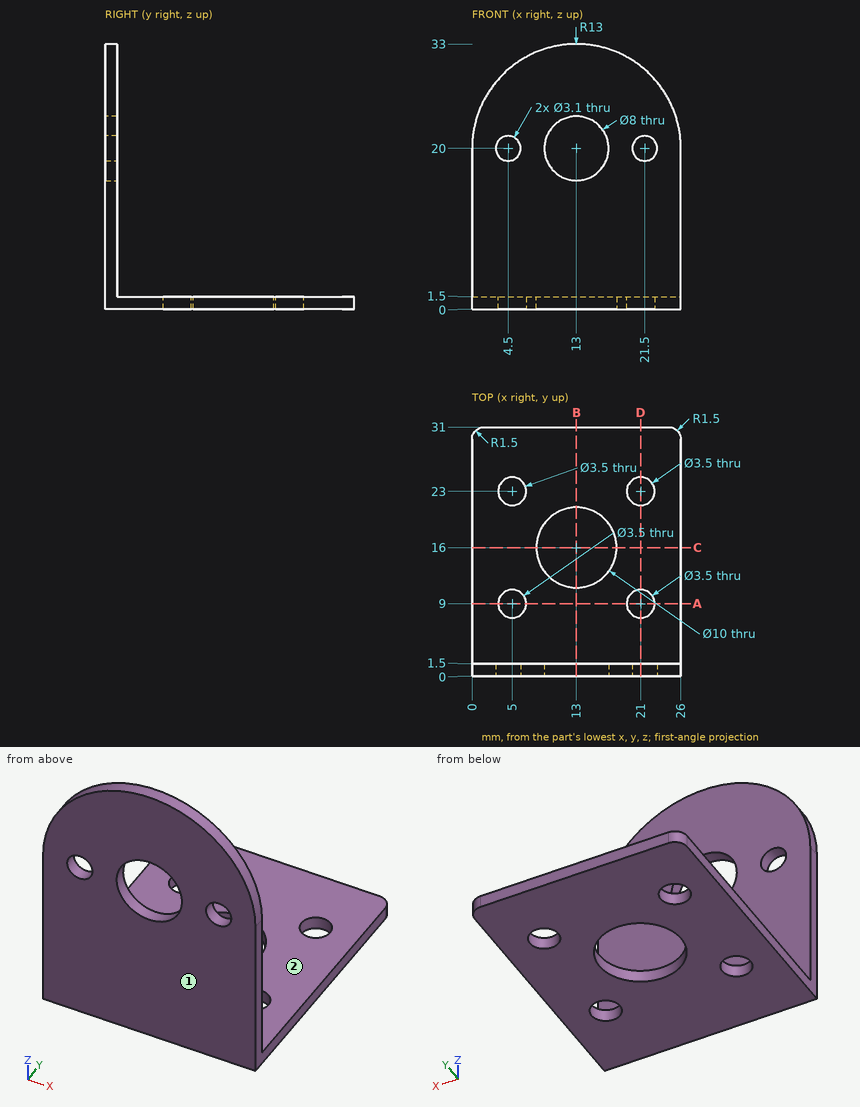
Here's the drawing with two shaded views (mm, measured from the low corner). I have some questions. A direction names the side the tool comes from. Coordinates: 2 decimals unless noted, no trailing zeros. Order: outer loops, then holes, each group sorted by start corner. A loop starts at its lowest first (then second) coordinate and runs counter-clockwise, first axis right, second up. Notation, with made-up numbers: (28, 56) - (34, 56) arc R34 ccw to (34, 94) - close; hole circle Ø8 at (44, 74). An arc over 180 degrees is marked (long way). Answer in a Markdown table with one row per item. Add a question column.
(1) If we section it at D-D, the plane x = 21: Please give me the cut outline in (y, z), then the cut area to 3 significant figures.
(2) I need wall thicknesses on L1, parallel to Y at x = 21, z = 1.2; L2, parallel to X at y = 0.5, z = 20; L3, parallel to Z at x = 12.5, y = 28. Which ranges of each line are inside material? Lowest first, please.
(3) On a 3-axis mill with a long thin cutter (end or side, diameter ignored), from which of +Z, -Z, +X, -X, +Y, -Y can I reach the whole of each face in a straight line? I mean the marked faces 1 and 2. Say none if no direction works.
(4) Will these pins go through, and if not, where does the flat tip stop? pin 1 (3 mm diameter, centred on x = 4, z = 19, fed in from +Y); pin 2 (4 mm diameter, centred on x = 21, y = 23, fed in from +Z).
(5) If we section it at C-C, the plane y = 16: Please give me the cut outline in (x, z), then the cut area to 3 significant figures.
(6) If we section it at B-B, the plane x = 13: Please give me the cut outline in (y, z), then the cut area to 4 significant figures.
(7) If we section it at A-A, the plane y = 9: Please give me the cut outline in (x, z), then the cut area to 3 significant figures.
Results are:
| question | item | result |
|---|---|---|
| 1 | outline | (0, 0) - (7.25, 0) - (7.25, 1.5) - (1.5, 1.5) - (1.5, 18.53) - (0, 18.53) - close; (0, 21.47) - (1.5, 21.47) - (1.5, 30.25) - (0, 30.25) - close; (10.75, 0) - (21.25, 0) - (21.25, 1.5) - (10.75, 1.5) - close; (24.75, 0) - (31, 0) - (31, 1.5) - (24.75, 1.5) - close |
| 1 | area | 74.7 mm2 |
| 2 | L1 | y = 0 to 7.25, 10.75 to 21.25, 24.75 to 31 |
| 2 | L2 | x = 0 to 2.95, 6.05 to 9, 17 to 19.95, 23.05 to 26 |
| 2 | L3 | z = 0 to 1.5 |
| 3 | face 1 | +Z, -Z, +X, -X, -Y |
| 3 | face 2 | +Z, +X, -X, +Y |
| 4 | pin 1 | stops at y = 1.5 |
| 4 | pin 2 | stops at z = 1.5 |
| 5 | outline | (0, 0) - (8, 0) - (8, 1.5) - (0, 1.5) - close; (18, 0) - (26, 0) - (26, 1.5) - (18, 1.5) - close |
| 5 | area | 24.0 mm2 |
| 6 | outline | (0, 0) - (11, 0) - (11, 1.5) - (1.5, 1.5) - (1.5, 16) - (0, 16) - close; (0, 24) - (1.5, 24) - (1.5, 33) - (0, 33) - close; (21, 0) - (31, 0) - (31, 1.5) - (21, 1.5) - close |
| 6 | area | 66.75 mm2 |
| 7 | outline | (0, 0) - (3.25, 0) - (3.25, 1.5) - (0, 1.5) - close; (6.75, 0) - (19.25, 0) - (19.25, 1.5) - (6.75, 1.5) - close; (22.75, 0) - (26, 0) - (26, 1.5) - (22.75, 1.5) - close |
| 7 | area | 28.5 mm2 |
